Geometry: final body of the model. Coordinates: model frame, mm. Face numbers are marked on the shaded views. A direction names the side the tool comes from. Give positions to 0.01 mm unless a question says otherwise; leave off trailing zeros. Write each loop counter-clockwise with the first axis right and the second up, starting at its lowest first coordinate (ties: lowest second). Pieces come first, ordered by that corner, then holes. Notation, with made-up numbers: M 31,-1.5 L 50,-1.5 A23 ccw 50,31.5 Z; hole C -14,5 d2. An arc over 180 degrees is marked long. One line per question, with ' | ' between items.
from build123d import *

# Parameters (mm, degrees)
F1_DEPTH = 101.6


with BuildPart() as f1:
    # F0 (on Front) → F1 (new body)
    with BuildSketch(Plane.XZ):
        Polygon((12.573, 25.032173), (10.980174, 28.448), (9.018368, 28.448), (10.795, 24.638), (0, 24.638), (0, 21.844), (10.795, 21.844), (10.795, 14.224), (4.191, 14.224), (4.191, 12.446), (10.795, 12.446), (7.936518, 1.778), (6.731, 1.778), (6.731, 0), (9.300825, 0), (12.573, 12.211922), align=None)
        Polygon((0, 21.844), (0, 24.638), (-10.795, 24.638), (-9.018368, 28.448), (-10.980174, 28.448), (-12.573, 25.032173), (-12.573, 12.211922), (-9.300825, 0), (-6.731, 0), (-6.731, 1.778), (-7.936518, 1.778), (-10.795, 12.446), (-4.191, 12.446), (-4.191, 14.224), (-10.795, 14.224), (-10.795, 21.844), align=None)
    extrude(amount=F1_DEPTH)


solid = f1.part
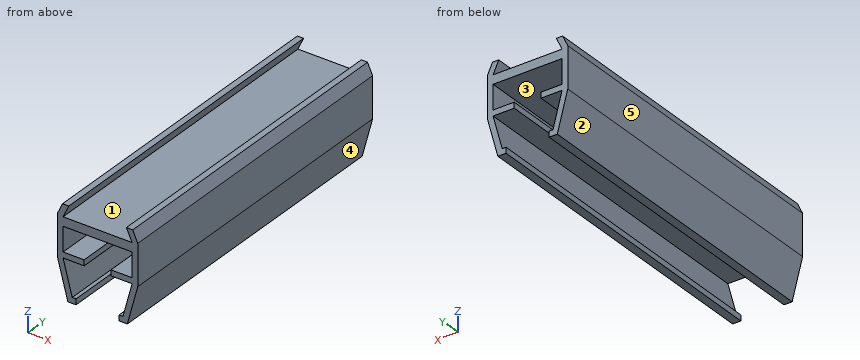
(1) Cut plane D-D, the plane z = 10.75. Return loops of the section in (x, y), then the cut area to 3 significant figures.
Working result:
outline: M -12.18,-101.6 L -10.34,-101.6 L -10.34,0 L -12.18,0 Z; M 10.34,-101.6 L 12.18,-101.6 L 12.18,0 L 10.34,0 Z | area: 374 mm^2
(2) Cut plane A-A, the plane z = 16. Return loops of the section in (x, y) (3 decimals).
Working result:
outline: M -12.573,-101.6 L -10.795,-101.6 L -10.795,0 L -12.573,0 Z; M 10.795,-101.6 L 12.573,-101.6 L 12.573,0 L 10.795,0 Z
(3) Set-up query: the marked faces 1 and 2. Return all of +Z, -Z, +X, -X, +Y, -Y with unobstructed straight access to the full face (end or side cutting, diameter ignored); none if empty.
Working result:
face 1: +Y, -Y | face 2: -Z, -X, +Y, -Y
(4) First-contact query: P1, Ø1.3, axis at x = -7.5, y = -28.5, coming from the +Z side; P2, Ø2, axis at y = -26.5, z = 1, coming from the +X side; P3, Ø0.9, axis at y = -55, z = 1, coming from the -X side. Flat tips, straight axial feed; report the tip coordinate or a pass-through.
Working result:
P1: stops at z = 24.64 | P2: stops at x = 9.84 | P3: stops at x = -9.69
(5) Cut plane B-B, the plane y = -11. Return loops of the section in (x, z) (3 decimals), then the cut area to 3 significant figures.
Working result:
outline: M -12.573,12.212 L -9.301,0 L -6.731,0 L -6.731,1.778 L -7.937,1.778 L -10.795,12.446 L -4.191,12.446 L -4.191,14.224 L -10.795,14.224 L -10.795,21.844 L 10.795,21.844 L 10.795,14.224 L 4.191,14.224 L 4.191,12.446 L 10.795,12.446 L 7.937,1.778 L 6.731,1.778 L 6.731,0 L 9.301,0 L 12.573,12.212 L 12.573,25.032 L 10.98,28.448 L 9.018,28.448 L 10.795,24.638 L -10.795,24.638 L -9.018,28.448 L -10.98,28.448 L -12.573,25.032 Z | area: 191 mm^2
(6) Draft query along X for the marked faces 3, 4 and 5. Return one class per face: released by +X, released by -X, zero draft, split by the parting line, or undercut.
Working result:
face 3: undercut | face 4: released by +X | face 5: released by -X
(7) Cut plane C-C, the plane x = 1. Return loops of the section in (y, z).
Working result:
outline: M -101.6,21.84 L 0,21.84 L 0,24.64 L -101.6,24.64 Z
(8) Material intervals for L1, parallel to Z at x = -7.25, y = -20; L2, parallel to Z at x = -6.25, y = -67; L3, parallel to X at y = -58, z = 21 (3 decimals), sorted ascending. Write a range as [from, to].
Working result:
L1: z = [0, 1.78], [12.45, 14.22], [21.84, 24.64] | L2: z = [12.45, 14.22], [21.84, 24.64] | L3: x = [-12.573, -10.795], [10.795, 12.573]
